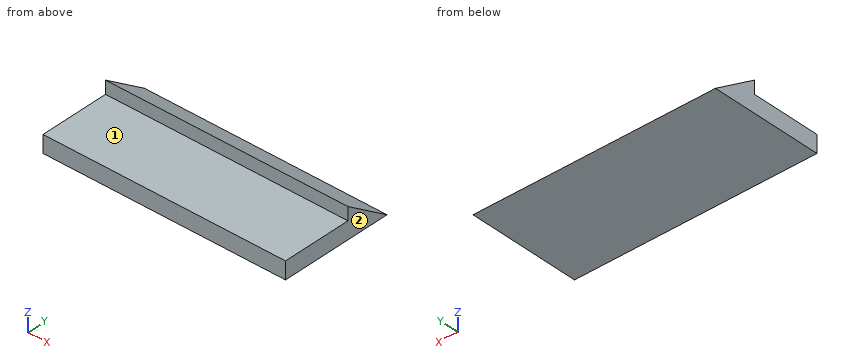
Autodesk Fusion 360 part; units mm, degrees
sketch "Esquisse1" plane through (0, 0, 0) normal (0, 0, 1) x (1, 0, 0)
  line L0 (0, 0) -> (28, 0)
  line L1 (28, 0) -> (28, 13)
  line L2 (28, 13) -> (0, 13)
  line L3 (0, 13) -> (0, 0)
  dimension "d1" = 28
  dimension "d2" = 13
extrude "Extrusion1" add sketch "Esquisse1" along normal blind 2
sketch "Esquisse2" plane through (0, 0, 2) normal (0, 0, 1) x (-1, 0, 0)
  line L0 (0, -13) -> (0, 0)
  line L1 (0, 0) -> (-28, 0)
  line L2 (-28, 0) -> (-28, -13)
  line L3 (-28, -13) -> (0, -13)
  line L4 (0, -13) -> (-28, -13)
  line L5 (-28, -13) -> (-28, -8)
  line L6 (-28, -8) -> (0, -8)
  line L7 (0, -8) -> (0, -13)
  dimension "d5" = 5
extrude "Extrusion2" add sketch "Esquisse2" along normal blind 1.5 contours L0 L2 L3 L4 L5 L6 L7
chamfer "Chanfrein1" distance 5 distance2 3.5 1 edges at (14, 13, 3.5) measured on face at (9.3333, 11.3333, 3.5)
The model under review builds one solid part; all positions refer to its coordinate system, in mm. Face numbers are marked on the shaded views. A direction names the side the tool comes from. Round coordinates to 2 decimals unless told otherwise and drop trailing zeros. Write each loop counter-clockwise with the first axis right and the second up, starting at its lowest first coordinate (ties: lowest second). Pieces come first, ordered by that corner, then holes. Notation, with made-up numbers: (26.5, -18.75) - (31.5, -18.75) arc R20 cw to (31.5, 17.25) - close; hole circle Ø1 at (53.25, -3.5). An arc over 180 degrees is marked (long way). One line per question, with ' | ' between items.
Item 1: For the marked faces 1 and 2, list the 3-axis set-ups (+Z, -Z, +X, -X, +Y, -Y) from which the entire face can be reached by the end or side of a thin tool; tool diameter is ignored.
Resolved:
face 1: +Z, +X, -X, -Y | face 2: +Z, -Z, +X, +Y, -Y
Item 2: For P1, Ø6.5, axis at x = 10.5, y = 3, coming from the +Z side; P2, Ø2, axis at x = 17, z = 1.5, coming from the +Y side, all flat-tipped, find the tip position at first contact; note any pin that passes through.
Resolved:
P1: stops at z = 2 | P2: stops at y = 12.29
Item 3: To check wall thickness, follow probe 1 along Z at (x, y) = (17.5, 2); probe 2 along Y at (x, z) = (17.25, 0.9); probe 3 along Z at (x, y) = (10.5, 10.75). State the ranges of each line that lie inside material, in increasing order.
Resolved:
probe 1: z = 0 to 2 | probe 2: y = 0 to 11.72 | probe 3: z = 0 to 1.58
Item 4: Add section B-B, the plane y = 2. Give the boundary of the cut face in (x, z).
Resolved:
outline: (0, 0) - (28, 0) - (28, 2) - (0, 2) - close
Item 5: Add section C-C, the plane z = 2.85. Give the boundary of the cut face in (x, y), then the cut area to 3 significant figures.
Resolved:
outline: (0, 8) - (28, 8) - (28, 8.93) - (0, 8.93) - close | area: 26.0 mm2
